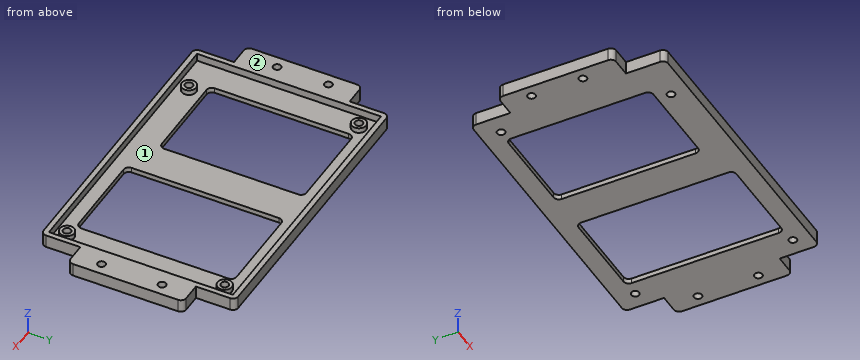
```python
from build123d import *

# Parameters (mm, degrees)
F0_W     = 106
F0_H     = 70
F0_R     = 2.75
F1_DEPTH = 2
F0_R_2   = 1.5
F2_DEPTH = 4
F0_W_2   = 9
F0_H_2   = 44
F3_DEPTH = 5
F4_R     = 2
F6_DEPTH = 2


with BuildPart() as f1:
    # F0 (on Top) → F1 (new body)
    with BuildSketch(Plane.XY):
        with Locations((-0.241208, 2.403659)):
            Rectangle(F0_W, F0_H)
        with Locations((-38.491208, -27.846341)):
            Circle(F0_R, mode=Mode.SUBTRACT)
        with Locations((48.258792, -28.096341)):
            Circle(F0_R, mode=Mode.SUBTRACT)
        with Locations((-47.741208, 31.903659)):
            Circle(F0_R, mode=Mode.SUBTRACT)
        with Locations((48.258792, 31.903659)):
            Circle(F0_R, mode=Mode.SUBTRACT)
    extrude(amount=F1_DEPTH)

    # F0 (on Top) → F2 (join)
    with BuildSketch(Plane.XY):
        with Locations((-47.741208, 31.903659)):
            Circle(F0_R)
        with Locations((-47.741208, 31.903659)):
            Circle(F0_R_2, mode=Mode.SUBTRACT)
        with Locations((-38.491208, -27.846341)):
            Circle(F0_R)
        with Locations((-38.491208, -27.846341)):
            Circle(F0_R_2, mode=Mode.SUBTRACT)
        with Locations((48.258792, -28.096341)):
            Circle(F0_R)
        with Locations((48.258792, -28.096341)):
            Circle(F0_R_2, mode=Mode.SUBTRACT)
        with Locations((48.258792, 31.903659)):
            Circle(F0_R)
        with Locations((48.258792, 31.903659)):
            Circle(F0_R_2, mode=Mode.SUBTRACT)
    extrude(amount=F2_DEPTH)

    # F0 (on Top) → F3 (join)
    with BuildSketch(Plane.XY):
        with Locations((-59.741208, 2.403659)):
            Rectangle(F0_W_2, F0_H_2)
        with Locations((-59.741208, -5.596341)):
            Circle(F0_R_2, mode=Mode.SUBTRACT)
        with Locations((-59.741208, 13.903659)):
            Circle(F0_R_2, mode=Mode.SUBTRACT)
        with BuildLine():
            ThreePointArc((-53.241208, 39.403659), (-54.655421, 38.817872), (-55.241208, 37.403659))
            Line((-55.241208, 37.403659), (-55.241208, 24.403659))
            Line((-55.241208, 24.403659), (-55.241208, -19.596341))
            Line((-55.241208, -19.596341), (-55.241208, -32.596341))
            ThreePointArc((-55.241208, -32.596341), (-54.655421, -34.010555), (-53.241208, -34.596341))
            Line((-53.241208, -34.596341), (52.758792, -34.596341))
            ThreePointArc((52.758792, -34.596341), (54.173006, -34.010555), (54.758792, -32.596341))
            Line((54.758792, -32.596341), (54.758792, -19.596341))
            Line((54.758792, -19.596341), (54.758792, 24.403659))
            Line((54.758792, 24.403659), (54.758792, 37.403659))
            ThreePointArc((54.758792, 37.403659), (54.173006, 38.817872), (52.758792, 39.403659))
            Line((52.758792, 39.403659), (-53.241208, 39.403659))
        make_face()
        with Locations((-0.241208, 2.403659)):
            Rectangle(F0_W, F0_H, mode=Mode.SUBTRACT)
        with Locations((59.258792, 2.403659)):
            Rectangle(F0_W_2, F0_H_2)
        with Locations((59.258792, -9.096341)):
            Circle(F0_R_2, mode=Mode.SUBTRACT)
        with Locations((59.258792, 13.903659)):
            Circle(F0_R_2, mode=Mode.SUBTRACT)
    extrude(amount=F3_DEPTH)

    # F4
    f4_edges = [f1.edges().sort_by_distance(p)[0] for p in [
        (-64.241208, 24.403659, 2.5),
        (-64.241208, -19.596341, 2.5),
        (63.758792, -19.596341, 2.5),
        (63.758792, 24.403659, 2.5),
    ]]
    fillet(f4_edges, radius=F4_R)

    # F5 (on face) → F6 (cut)
    with BuildSketch(Plane.XY.offset(2)):
        with BuildLine():
            Line((8.758792, -27.596341), (40.758792, -27.596341))
            ThreePointArc((40.758792, -27.596341), (42.173006, -27.010555), (42.758792, -25.596341))
            Line((42.758792, -25.596341), (42.758792, 30.403659))
            ThreePointArc((42.758792, 30.403659), (42.173006, 31.817872), (40.758792, 32.403659))
            Line((40.758792, 32.403659), (8.758792, 32.403659))
            ThreePointArc((8.758792, 32.403659), (7.344579, 31.817872), (6.758792, 30.403659))
            Line((6.758792, 30.403659), (6.758792, -25.596341))
            ThreePointArc((6.758792, -25.596341), (7.344579, -27.010555), (8.758792, -27.596341))
        make_face()
        with BuildLine():
            Line((-41.241208, -22.596341), (-9.241208, -22.596341))
            ThreePointArc((-9.241208, -22.596341), (-7.826994, -22.010555), (-7.241208, -20.596341))
            Line((-7.241208, -20.596341), (-7.241208, 30.403659))
            ThreePointArc((-7.241208, 30.403659), (-7.826994, 31.817872), (-9.241208, 32.403659))
            Line((-9.241208, 32.403659), (-41.241208, 32.403659))
            ThreePointArc((-41.241208, 32.403659), (-42.655421, 31.817872), (-43.241208, 30.403659))
            Line((-43.241208, 30.403659), (-43.241208, -20.596341))
            ThreePointArc((-43.241208, -20.596341), (-42.655421, -22.010555), (-41.241208, -22.596341))
        make_face()
    extrude(amount=-F6_DEPTH, mode=Mode.SUBTRACT)


solid = f1.part
```
Check sheet for the modelled part. Datum: model origin and axes. Units: mm. Face numbers are marked on the shaded views. Coordinates: 2 decimals unless noted, no trailing zeros. Order: outer loops, then holes, each group sorted by start corner. A loop starts at its lowest first (then second) coordinate and runs counter-clockwise, first axis right, second up. Notation, with made-up numbers: (70.5, -24.5) -> (75.5, -24.5) arc R22 cw to (75.5, -14.5) -> close; hole circle Ø9 at (80.25, 8.25). An arc over 180 degrees is marked (long way). Write each question's results on one line, items separated by ' | '. Start each with the question number.
1) Section check B-B (y = -16). Enter the section's corners in (x, z), and give its area (3 significant figures).
2) Depth check by flat-ended pin: pin 1 (1.5 mm diameter, centred on x = 57.5, z = 2.5, fed in from -Y); pin 2 (4.5 mm diameter, centred on x = 48.5, y = 32.5, fed in from +Z); pin 3 (1.5 mm diameter, centred on x = -60, z = 3.5, fed in from +Y); pin 4 (8 mm diameter, centred on x = -38.5, y = -15, fed in from +Z). Enter the tip coordinate at first touch or a pass-through.
3) Section check C-C (x = -1). Enter the section's corners in (y, z).
4) Draft check along Y on the marked faces 1 and 2. Enter one of: pulls with the +Y half, pulls with the -Y half, needs draft (parallel to the pull), parting line crosses it, or undercut.
5) Material ranges on line 1 along X through (y, z) = (28, 1.85); line 2 along X through (y, z) = (32, 2.6); line 3 along X through (y, z) = (17, 1.8), recorded low to high.
6) Section check A-A (x = 15). Enter the section's corners in (y, z), and give its area (3 significant figures).
7) Section check D-D (x = -27.5). Enter the section's corners in (y, z), and give its area (3 significant figures).
Checked values:
1) outline: (-64.24, 0) -> (-43.24, 0) -> (-43.24, 2) -> (-53.24, 2) -> (-53.24, 5) -> (-64.24, 5) -> close; (-7.24, 0) -> (6.76, 0) -> (6.76, 2) -> (-7.24, 2) -> close; (42.76, 0) -> (63.76, 0) -> (63.76, 5) -> (52.76, 5) -> (52.76, 2) -> (42.76, 2) -> close | area: 178 mm²
2) pin 1: y = -19.6 | pin 2: z = 4 | pin 3: y = 24.4 | pin 4: through
3) outline: (-34.6, 0) -> (39.4, 0) -> (39.4, 5) -> (37.4, 5) -> (37.4, 2) -> (-32.6, 2) -> (-32.6, 5) -> (-34.6, 5) -> close
4) face 1: undercut | face 2: needs draft
5) line 1: -55.24 to -43.24, -7.24 to 6.76, 42.76 to 54.76 | line 2: -55.24 to -53.24, -50.49 to -49.24, -46.24 to -44.99, 45.51 to 46.76, 49.76 to 51.01, 52.76 to 54.76 | line 3: -64.24 to -43.24, -7.24 to 6.76, 42.76 to 63.76
6) outline: (-34.6, 0) -> (-27.6, 0) -> (-27.6, 2) -> (-32.6, 2) -> (-32.6, 5) -> (-34.6, 5) -> close; (32.4, 0) -> (39.4, 0) -> (39.4, 5) -> (37.4, 5) -> (37.4, 2) -> (32.4, 2) -> close | area: 40.0 mm²
7) outline: (-34.6, 0) -> (-22.6, 0) -> (-22.6, 2) -> (-32.6, 2) -> (-32.6, 5) -> (-34.6, 5) -> close; (32.4, 0) -> (39.4, 0) -> (39.4, 5) -> (37.4, 5) -> (37.4, 2) -> (32.4, 2) -> close | area: 50.0 mm²
